Can you work these out from the model? Positions are in its coordinate system, mm. A direction names the side the tool comes from. Coordinates: 2 decimals unless noted, no trailing zeros. Loops run counter-clockwise (first coordinate to the right, second up) from the corner with the lowest first, then second, coordinate; pieces in that order, holes last.
```python
from build123d import *

# Parameters (mm, degrees)
BOSS_EXTRUDE2_DEPTH     = 75
CUT_EXTRUDE1_DEPTH      = 148
CUT_EXTRUDE1_DEPTH_BACK = 47
SKETCH2_R               = 5
FILLET1_R               = 37.5
FILLET2_R               = 10


with BuildPart() as part:
    # Sketch1 → Boss-Extrude2 (new body)
    with BuildSketch(Plane.XY):
        Polygon((8, -117), (8, -8), (67, -8), (67, -117), (67, -121), (67, -129), (95.5, -129), (95.5, -250), (103.5, -250), (103.5, -121), (75, -121), (75, -8), (75, 0), (67, 0), (8, 0), (0, 0), (0, -8), (0, -121), (-28.5, -121), (-28.5, -250), (-20.5, -250), (-20.5, -129), (8, -129), (8, -125), (8, -121), align=None)
    extrude(amount=BOSS_EXTRUDE2_DEPTH)

    # Sketch2 → Cut-Extrude1 (cut, two sides: drawn at the far end of the back side and taken through both)
    with BuildSketch(Plane(origin=(0, 0, 0), x_dir=(0, 0, -1), z_dir=(1, 0, 0)).offset(-CUT_EXTRUDE1_DEPTH_BACK)):
        with Locations(Location((-37.5, -212.5, 0), (0, 0, 90))):
            Circle(SKETCH2_R)
    extrude(amount=CUT_EXTRUDE1_DEPTH + CUT_EXTRUDE1_DEPTH_BACK, mode=Mode.SUBTRACT)

    # Fillet1
    fillet1_edges = [part.edges().sort_by_distance(p)[0] for p in [
        (-24.5, -250, 0),
        (-24.5, -250, 75),
        (99.5, -250, 0),
        (99.5, -250, 75),
    ]]
    fillet(fillet1_edges, radius=FILLET1_R - 0.0001)  # a hair under: the kernel refuses the full size

    # Fillet2
    fillet2_edges = [part.edges().sort_by_distance(p)[0] for p in [
        (0, -121, 37.5),
        (75, -121, 37.5),
    ]]
    fillet(fillet2_edges, radius=FILLET2_R)


solid = part.part
```
(1) I want a section at C-C on x = 21. Write out the boundary of the cut face in (y, z).
Check values:
outline: (-8, 0) - (0, 0) - (0, 75) - (-8, 75) - close
(2) If we mould it in two halves opening along Y, with no side actions, what happens to faces 4 (the cylindrical face through (78.01, -118.15, 38.02)), 5 (the flat face through (103.5, -186, 37)), 6 (the cylindrical face through (-24.56, -207.73, 39)), 7 (the cylindrical face through (99.44, -207.73, 39))? For each: released by +Y, released by -Y, zero draft, split by the parting line, or undercut.
Check values:
face 4: released by +Y
face 5: zero draft
face 6: undercut
face 7: undercut
(3) I want a section at D-D on z = 12.5. Write out the boundary of the cut face in (x, y).
Check values:
outline: (-28.5, -240.45) - (-20.5, -240.45) - (-20.5, -129) - (8, -129) - (8, -8) - (67, -8) - (67, -129) - (95.5, -129) - (95.5, -240.45) - (103.5, -240.45) - (103.5, -121) - (85, -121) arc R10 cw to (75, -111) - (75, 0) - (0, 0) - (0, -111) arc R10 cw to (-10, -121) - (-28.5, -121) - close
(4) I want a section at A-A on y = -107. Write out the boundary of the cut face in (x, z), then the cut area to 3 significant figures.
Check values:
outline: (0, 0) - (8, 0) - (8, 75) - (0, 75) - close; (67, 0) - (75, 0) - (75, 75) - (67, 75) - close
area: 1,200 mm2
(5) I'm going to push flat-ended pins straight in: pin 1 (12 mm diameter, centred on x = -13, z = 54, fed in from -Y); pin 2 (8 mm diameter, centred on y = -101, z = 54, fed in from -X); pin 3 (1 mm diameter, centred on x = -15, z = 32.5, fed in from +Y). Where does each tip first touch, or does it pass through?
Check values:
pin 1: stops at y = -129
pin 2: stops at x = 0
pin 3: stops at y = -121
(6) I want a section at B-B on z = 60.5. Write out the boundary of the cut face in (x, y), then the cut area to 3 significant figures.
Check values:
outline: (-28.5, -242.12) - (-20.5, -242.12) - (-20.5, -129) - (8, -129) - (8, -8) - (67, -8) - (67, -129) - (95.5, -129) - (95.5, -242.12) - (103.5, -242.12) - (103.5, -121) - (85, -121) arc R10 cw to (75, -111) - (75, 0) - (0, 0) - (0, -111) arc R10 cw to (-10, -121) - (-28.5, -121) - close
area: 4,840 mm2
(7) Which directions (+Z, -Z, +X, -X, +Y, -Y) give clear straight access to the entire face, cutting with the end or side of a thin tool? Please do faces 1 (the flat face through (37, -8, 37)), 2 (the flat face through (3, -98, 75)), 3 (the flat face through (94, -121, 37)).
Check values:
face 1: +Z, -Z, -Y
face 2: +Z, +X, -X, +Y, -Y
face 3: +Z, -Z, +X, +Y
(8) If I drill on probe 1 along Y at (x, z) = (98.25, 37.5); probe 2 along X at (y, z) = (-61.5, 70); probe 3 along Z at (x, y) = (-25.75, -212.5), over which ranges is the centre line in solid material (lowest first)?
Check values:
probe 1: y = -250 to -217.5, -207.5 to -121
probe 2: x = 0 to 8, 67 to 75
probe 3: z = 0 to 32.5, 42.5 to 75
